For this review, use the dimensioned drawing (mm, ordinates from the lowest corner) and the shaded views. A direction names the side the tool comes from. Give positions to 0.01 mm unless a question says otherwise; leave off trailing zeros. Order: outer loops, then holes, each group sorted by start corner. A loop starts at its lowest first (then second) coordinate and runs counter-clockwise, first axis right, second up.
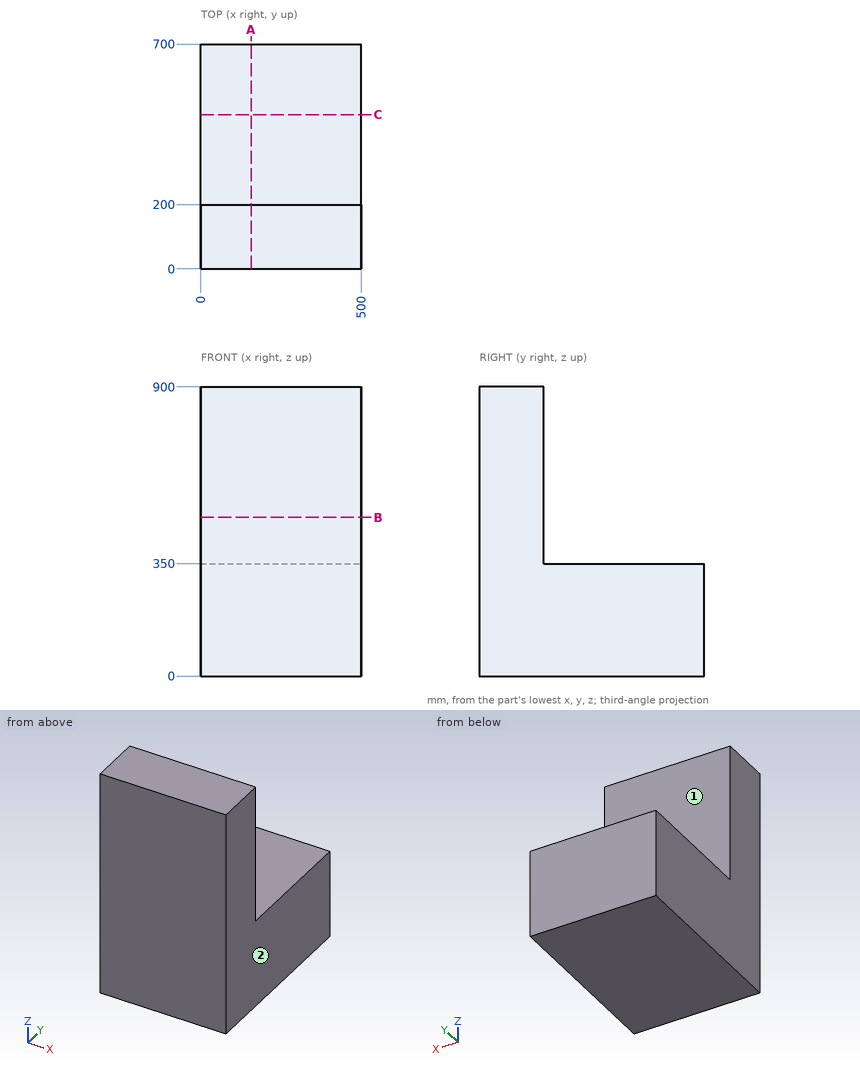
1. For the marked faces 1 and 2, list the 3-axis set-ups (+Z, -Z, +X, -X, +Y, -Y) from which the entire face can be reached by the end or side of a thin tool; tool diameter is ignored.
2. Take a section at A-A (x = 156.5). Write out the cut boundary in (y, z), and give its area (3 significant figures).
3. Take a section at C-C (y = 480). Write out the cut boundary in (x, z).
4. Insertion check: pin 1 (1 mm diameter, centred on x = 312.5, y = 365.5, fed in from +Z). The pin has a flat end and moves straight along its axis. Give the tip position at first contact, or say it passes through.
5. Take a section at B-B (z = 493.5). Write out the cut boundary in (x, y).
6. To check wall thickness, follow line 1 (Y direction, x = 351.5, z = 699); line 2 (Z direction, x = 58.5, y = 355). State the ranges of each line that lie inside material, in increasing order.
Answer:
1. face 1: +Z, +X, -X, +Y
1. face 2: +Z, -Z, +X, +Y, -Y
2. outline: (0, 0) - (700, 0) - (700, 350) - (200, 350) - (200, 900) - (0, 900) - close
2. area: 355,000 mm2
3. outline: (0, 0) - (500, 0) - (500, 350) - (0, 350) - close
4. pin 1: stops at z = 350
5. outline: (0, 0) - (500, 0) - (500, 200) - (0, 200) - close
6. line 1: y = 0 to 200
6. line 2: z = 0 to 350
